Input: part model. Units: mm. Frame: model coordinates. Round coordinates to 2 decimals unless told otherwise and drop trailing zeros. Loops run counter-clockwise (first coordinate to the right, second up) from the corner with the lowest first, then second, coordinate; pieces in that order, holes last. Notation, with made-up numbers: M -1,-37 L 8,-37 A26 cw 8,-5 Z; hole C 21,59.25 d1. An arc over 180 degrees is marked long. Use one line per item in the form item = value. Start each with the question number.
Q1. Section query D-D, the plane y = 6. Output: boundary loops of the cut face in (x, z).
Q2. First-contact query: P1, Ø6, axis at y = 5.5, z = 1.5, coming from the +X side; P2, Ø2, axis at x = 0, y = 14, coming from the +Z side; P3, Ø4, axis at x = 4.5, z = 3.5, coming from the +Y side. Flat tips, straight axial feed; report the tip coordinate or a pass-through.
Q3. Section query B-B, the plane z = 8. Output: boundary loops of the cut face in (x, y).
Q4. Ray query, line 1 along Y through (x, z) = (0, 4); line 2 along Y through (x, z) = (-0.5, 4.5); line 3 along Y through (x, z) = (-13.5, 3.75). Return the intervals inside material, ascending.
Q5. Section query A-A, the plane x = 0. Output: boundary loops of the cut face in (y, z), and give its area (3 significant figures).
Q6. Section query C-C, the plane x = -15. Output: boundary loops of the cut face in (y, z).
```python
from build123d import *

# Parameters (mm, degrees)
SKETCH_1_R      = 1.75
SKETCH_1_R_2    = 2.5
EXTRUDE_1_DEPTH = 10


with BuildPart() as part:
    # Эскиз1 → Бобышка-Вытянуть1 (new body)
    with BuildSketch(Plane.XY):
        with BuildLine():
            Line((-28.5, 0), (-28.5, -28.5))
            Line((-28.5, -28.5), (28.5, -28.5))
            Line((28.5, -28.5), (28.5, 0))
            ThreePointArc((28.5, 0), (0, 28.5), (-28.5, 0))
        make_face()
        with Locations((0, 14)):
            Circle(SKETCH_1_R, mode=Mode.SUBTRACT)
        with Locations((14, 0)):
            Circle(SKETCH_1_R, mode=Mode.SUBTRACT)
        with Locations((0, -14)):
            Circle(SKETCH_1_R, mode=Mode.SUBTRACT)
        with Locations((-14, 0)):
            Circle(SKETCH_1_R, mode=Mode.SUBTRACT)
        Circle(SKETCH_1_R_2, mode=Mode.SUBTRACT)
    extrude(amount=EXTRUDE_1_DEPTH)


solid = part.part
```
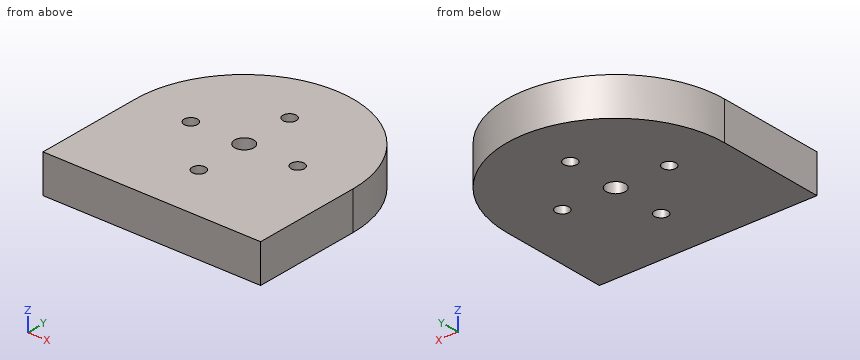
Results found:
q1.outline = M -27.86,0 L 27.86,0 L 27.86,10 L -27.86,10 Z
q2.P1 = 28.39
q2.P2 = through
q2.P3 = 28.39
q3.outline = M -28.5,-28.5 L 28.5,-28.5 L 28.5,0 A28.5 ccw -28.5,0 Z; hole C -14,0 d3.5; hole C 0,0 d5; hole C 0,-14 d3.5; hole C 0,14 d3.5; hole C 14,0 d3.5
q4.line_1 = -28.5 to -15.75, -12.25 to -2.5, 2.5 to 12.25, 15.75 to 28.5
q4.line_2 = -28.5 to -15.68, -12.32 to -2.45, 2.45 to 12.32, 15.68 to 28.5
q4.line_3 = -28.5 to -1.68, 1.68 to 25.1
q5.outline = M -28.5,0 L -15.75,0 L -15.75,10 L -28.5,10 Z; M -12.25,0 L -2.5,0 L -2.5,10 L -12.25,10 Z; M 2.5,0 L 12.25,0 L 12.25,10 L 2.5,10 Z; M 15.75,0 L 28.5,0 L 28.5,10 L 15.75,10 Z
q5.area = 450 mm²
q6.outline = M -28.5,0 L -1.44,0 L -1.44,10 L -28.5,10 Z; M 1.44,0 L 24.23,0 L 24.23,10 L 1.44,10 Z
